Build history of the part. All positions in model axes, mm. A direction names the side the tool comes from. Give positions to 0.01 mm unless a question says otherwise; leave off trailing zeros. Write each loop counter-clockwise with the first axis right and the second up, starting at its lowest first coordinate (ties: lowest second). Pieces come first, ordered by that corner, then holes.
from build123d import *

# Parameters (mm, degrees)
F0_W     = 12.7
F0_H     = 76.2
F1_DEPTH = 25.4
F0_W_2   = 177.8
F2_DEPTH = 25.4
F3_R     = 3.96875
F4_DEPTH = 254
F5_R     = 3.96875
F6_DEPTH = 152.4
F7_W     = 76.2
F7_H     = 15.875
F8_DEPTH = 25.4


with BuildPart() as f1:
    # F0 (on Top) → F1 (new body, symmetric)
    with BuildSketch(Plane.XY):
        Polygon((154.0158234471, 53.3519236594), (-74.5841765529, 53.3519236594), (-74.5841765529, 40.6519236594), (103.2158234471, 40.6519236594), (103.2158234471, -35.5480763406), (-74.5841765529, -35.5480763406), (-74.5841765529, -48.2480763406), (154.0158234471, -48.2480763406), align=None)
        with Locations((141.3158234471, 2.5519236594)):
            Rectangle(F0_W, F0_H, mode=Mode.SUBTRACT)
    extrude(amount=F1_DEPTH, both=True)

    # F0 (on Top) → F2 (join)
    with BuildSketch(Plane.XY):
        with Locations((14.3158234471, 2.5519236594)):
            Rectangle(F0_W_2, F0_H)
    extrude(amount=-F2_DEPTH)

    # F3 (on face) → F4 (cut)
    with BuildSketch(Plane.XZ.offset(48.2480763406)):
        with Locations((141.3158234471, 12.7)):
            Circle(F3_R)
    extrude(amount=-F4_DEPTH, mode=Mode.SUBTRACT)

    # F5 (on face) → F6 (cut)
    with BuildSketch(Plane.XZ.offset(48.2480763406)):
        with Locations((-61.8841765529, -12.7)):
            Circle(F5_R)
    extrude(amount=-F6_DEPTH, mode=Mode.SUBTRACT)

    # F7 (on face) → F8 (cut)
    with BuildSketch(Plane(origin=(-74.5841765529, 0, 0), x_dir=(0, -1, 0), z_dir=(-1, 0, 0))):
        with Locations((-2.5519236594, -17.4625)):
            Rectangle(F7_W, F7_H)
    extrude(amount=-F8_DEPTH, mode=Mode.SUBTRACT)


solid = f1.part
1. Saw through at D-D on z = -3. Give the cut face in (x, y).
2. Saw through at B-B on y = 29.5. Give the cut face in (x, z) (1 decimal).
3. Saw through at C-C on z = -12.7. Give the cut face in (x, y), plus the area to 3 significant figures.
4. Mould opens along X. For faces 1 (the face through (-49.184, 3, -17)), 2 (the face through (-59.751, 1.841, -9.354)), 3 (the face through (-62, 40.652, -18)) say: pulls with the +X half, pulls with the -X half, needs draft (parallel to the pull), parting line crosses it, or undercut.
5. Saw through at A-A on z = 12.7. Give the cut face in (x, y), plus the area to 3 significant figures.
6. 3-axis set-ups, long thin cutter, end or side, ignore diameter. For faces 4 (the face through (38, 3, -25.4)), 5 (the face through (-54, 3, -9.525)), 6 (the face through (103.216, 3, 13)), 7 (the face through (147.666, 2, 0)): which of +Z, -Z, +X, -X, +Y, -Y reach the whole face in a straight line?
7. Drop flat-ended pins along their axis: pin 1 (17.5 mm diameter, centred on y = -14, z = -17.5, fed in from -X); pin 2 (2 mm diameter, centred on x = -28, y = -26.5, fed in from +Z); pin 3 (3 mm diameter, centred on x = -68.5, y = -4, fed in from -Z) (3 decimals); pin 4 (6 mm diameter, centred on y = -25.5, z = 8, fed in from -X). Give the stop position or say it passes through.
8. Drill centre lines: line 1 along X through (y, z) = (10, -5.5); line 2 along X through (y, z) = (17.5, -21); line 3 along Y through (x, z) = (78.5, 11). Where is each one in solid material? Low to high.
Outcome:
1. outline: (-74.58, -48.25) - (154.02, -48.25) - (154.02, 53.35) - (-74.58, 53.35) - close; hole (134.97, -35.55) - (147.67, -35.55) - (147.67, 40.65) - (134.97, 40.65) - close
2. outline: (-74.6, -9.5) - (-64.3, -9.5) arc R4 cw to (-59.5, -9.5) - (-49.2, -9.5) - (-49.2, -25.4) - (135, -25.4) - (135, 25.4) - (103.2, 25.4) - (103.2, 0) - (-74.6, 0) - close; (147.7, -25.4) - (154, -25.4) - (154, 25.4) - (147.7, 25.4) - close
3. outline: (-74.58, -48.25) - (-65.85, -48.25) - (-65.85, -35.55) - (-74.58, -35.55) - close; (-74.58, 40.65) - (-65.85, 40.65) - (-65.85, 53.35) - (-74.58, 53.35) - close; (-57.92, -48.25) - (154.02, -48.25) - (154.02, 53.35) - (-57.92, 53.35) - (-57.92, 40.65) - (-49.18, 40.65) - (-49.18, -35.55) - (-57.92, -35.55) - close; hole (134.97, -35.55) - (147.67, -35.55) - (147.67, 40.65) - (134.97, 40.65) - close
3. area: 20,100 mm2
4. face 1: pulls with the -X half
4. face 2: undercut
4. face 3: needs draft
5. outline: (-74.58, -48.25) - (137.35, -48.25) - (137.35, -35.55) - (134.97, -35.55) - (134.97, 40.65) - (137.35, 40.65) - (137.35, 53.35) - (-74.58, 53.35) - (-74.58, 40.65) - (103.22, 40.65) - (103.22, -35.55) - (-74.58, -35.55) - close; (145.28, -48.25) - (154.02, -48.25) - (154.02, 53.35) - (145.28, 53.35) - (145.28, 40.65) - (147.67, 40.65) - (147.67, -35.55) - (145.28, -35.55) - close
5. area: 8,510 mm2
6. face 4: -Z, +X, -X, +Y, -Y
6. face 5: -Z, -X
6. face 6: +Z, -X
6. face 7: +Z, -Z
7. pin 1: stops at x = -74.58
7. pin 2: stops at z = 0
7. pin 3: stops at z = -9.525
7. pin 4: stops at x = 103.22
8. line 1: x = -74.58 to 134.97, 147.67 to 154.02
8. line 2: x = -49.18 to 134.97, 147.67 to 154.02
8. line 3: y = -48.25 to -35.55, 40.65 to 53.35
